from build123d import *

# Parameters (mm, degrees)
BOSS_EXTRUDE1_DEPTH = 2
BOSS_EXTRUDE2_DEPTH = 10
SKETCH7_R           = 3
SKETCH7_R_2         = 1.100094
SKETCH7_R_3         = 1.100095
SKETCH7_R_4         = 1.14540164
SKETCH7_R_5         = 1.100094267
BOSS_EXTRUDE3_DEPTH = 4
CUT_EXTRUDE1_DEPTH  = 3
FILLET2_R           = 1.3
CHAMFER1_SIZE       = 0.75
CHAMFER2_SIZE       = 0.5


with BuildPart() as part:
    # Sketch3 → Boss-Extrude1 (new body)
    with BuildSketch(Plane.XY):
        with BuildLine():
            Line((60.855233133, 23.823211938), (47.949977192, 24.377676222))
            Line((47.949977192, 24.377676222), (9.438001399, 18.932389733))
            ThreePointArc((9.438001399, 18.932389733), (7.157815869, 19.520564151), (5.962231275, 21.549300871))
            Line((5.962231275, 21.549300871), (-1.970708405, 77.995680607))
            ThreePointArc((-1.970708405, 77.995680607), (-1.383464331, 80.271537635), (0.639738461, 81.467794829))
            Line((0.639738461, 81.467794829), (38.699898469, 86.902208152))
            Line((38.699898469, 86.902208152), (38.171393284, 94.460167157))
            ThreePointArc((38.171393284, 94.460167157), (38.910984807, 96.683773594), (41.002517903, 97.740613468))
            Line((41.002517903, 97.740613468), (60.921819416, 99.276682226))
            Line((60.921819416, 99.276682226), (60.921819416, 103.721902307))
            ThreePointArc((60.921819416, 103.721902307), (61.804499235, 105.878127499), (63.945786912, 106.796450874))
            Line((63.945786912, 106.796450874), (83.059551455, 107.113531682))
            ThreePointArc((83.059551455, 107.113531682), (85.251859467, 106.245869167), (86.185286941, 104.080744272))
            Line((86.185286941, 104.080744272), (86.24375422, 99.780452187))
            Line((86.24375422, 99.780452187), (154.596820419, 99.780452187))
            ThreePointArc((154.596820419, 99.780452187), (156.771169517, 98.879807301), (157.671814403, 96.705458202))
            Line((157.671814403, 96.705458202), (157.671814403, 14.057773112))
            ThreePointArc((157.671814403, 14.057773112), (157.497078938, 13.035997261), (156.992732263, 12.130352296))
            Line((156.992732263, 12.130352296), (146.547659954, -0.852593653))
            ThreePointArc((146.547659954, -0.852593653), (144.453525054, -1.98521487), (142.178510717, -1.283401812))
            Line((142.178510717, -1.283401812), (127.110775499, 11.324099062))
            Line((127.110775499, 11.324099062), (110.204782414, 17.079131321))
            Line((110.204782414, 17.079131321), (91.635796855, 16.870620568))
            Line((91.635796855, 16.870620568), (72.085555936, 14.46343429))
            ThreePointArc((72.085555936, 14.46343429), (70.725838171, 14.602041008), (69.560483965, 15.316179508))
            Line((69.560483965, 15.316179508), (60.855233133, 23.823211938))
        make_face()
    extrude(amount=BOSS_EXTRUDE1_DEPTH)

    # Sketch4 → Boss-Extrude2 (add)
    with BuildSketch(Plane.XY):
        with BuildLine():
            Line((47.949977192, 24.377676222), (60.855233133, 23.823211938))
            Line((60.855233133, 23.823211938), (69.560483965, 15.316179508))
            ThreePointArc((69.560483965, 15.316179508), (70.725838171, 14.602041008), (72.085555936, 14.46343429))
            Line((72.085555936, 14.46343429), (91.635796855, 16.870620568))
            Line((91.635796855, 16.870620568), (110.204782414, 17.079131321))
            Line((110.204782414, 17.079131321), (127.110775499, 11.324099062))
            Line((127.110775499, 11.324099062), (142.178510717, -1.283401812))
            ThreePointArc((142.178510717, -1.283401812), (144.453525054, -1.98521487), (146.547659954, -0.852593653))
            Line((146.547659954, -0.852593653), (156.992732263, 12.130352296))
            ThreePointArc((156.992732263, 12.130352296), (157.497078938, 13.035997261), (157.671814403, 14.057773112))
            Line((157.671814403, 14.057773112), (157.671814403, 96.705458202))
            ThreePointArc((157.671814403, 96.705458202), (156.771169517, 98.879807301), (154.596820419, 99.780452187))
            Line((154.596820419, 99.780452187), (86.24375422, 99.780452187))
            Line((86.24375422, 99.780452187), (86.185286941, 104.080744272))
            ThreePointArc((86.185286941, 104.080744272), (85.251859467, 106.245869167), (83.059551455, 107.113531682))
            Line((83.059551455, 107.113531682), (63.945786912, 106.796450874))
            ThreePointArc((63.945786912, 106.796450874), (61.804499235, 105.878127499), (60.921819416, 103.721902307))
            Line((60.921819416, 103.721902307), (60.921819416, 99.276682226))
            Line((60.921819416, 99.276682226), (41.002517903, 97.740613468))
            ThreePointArc((41.002517903, 97.740613468), (38.910984807, 96.683773594), (38.171393284, 94.460167157))
            Line((38.171393284, 94.460167157), (38.699898469, 86.902208152))
            Line((38.699898469, 86.902208152), (0.639738461, 81.467794829))
            ThreePointArc((0.639738461, 81.467794829), (-1.383464331, 80.271537635), (-1.970708405, 77.995680607))
            Line((-1.970708405, 77.995680607), (5.962231275, 21.549300871))
            ThreePointArc((5.962231275, 21.549300871), (7.157815869, 19.520564151), (9.438001399, 18.932389733))
            Line((9.438001399, 18.932389733), (47.949977192, 24.377676222))
        make_face()
        with BuildLine():
            ThreePointArc((84.258355662, 98.692914663), (84.533669024, 98.04695842), (85.183308419, 97.780452187))
            Line((85.183308419, 97.780452187), (154.596820419, 97.780452187))
            ThreePointArc((154.596820419, 97.780452187), (155.356955955, 97.465593738), (155.671814403, 96.705458202))
            Line((155.671814403, 96.705458202), (155.671814403, 14.057773112))
            ThreePointArc((155.671814403, 14.057773112), (155.610734868, 13.70060696), (155.434438315, 13.38403486))
            Line((155.434438315, 13.38403486), (144.989366006, 0.401088911))
            ThreePointArc((144.989366006, 0.401088911), (144.257272174, 0.005133041), (143.461944249, 0.250481615))
            Line((143.461944249, 0.250481615), (128.108249423, 13.097251096))
            Line((128.108249423, 13.097251096), (110.524936275, 19.082852408))
            Line((110.524936275, 19.082852408), (91.501949272, 18.869243682))
            Line((91.501949272, 18.869243682), (71.841145237, 16.448443965))
            ThreePointArc((71.841145237, 16.448443965), (71.365754809, 16.496904248), (70.958318613, 16.74658445))
            Line((70.958318613, 16.74658445), (61.958856362, 25.54112911))
            ThreePointArc((61.958856362, 25.54112911), (61.679828995, 25.728441638), (61.352295386, 25.803701118))
            Line((61.352295386, 25.803701118), (47.852081394, 26.383727313))
            Line((47.852081394, 26.383727313), (9.158002316, 20.91269287))
            ThreePointArc((9.158002316, 20.91269287), (8.360780393, 21.118336461), (7.942767807, 21.827644264))
            Line((7.942767807, 21.827644264), (0.009828128, 78.274024))
            ThreePointArc((0.009828128, 78.274024), (0.215128769, 79.069664055), (0.922440855, 79.487875801))
            Line((0.922440855, 79.487875801), (39.972806225, 85.063675424))
            ThreePointArc((39.972806225, 85.063675424), (40.561555536, 85.398058084), (40.76480024, 86.043913413))
            Line((40.76480024, 86.043913413), (40.166521363, 94.599680421))
            ThreePointArc((40.166521363, 94.599680421), (40.425084652, 95.377059525), (41.156290542, 95.746533736))
            Line((41.156290542, 95.746533736), (62.067941403, 97.359127107))
            ThreePointArc((62.067941403, 97.359127107), (62.675544492, 97.652931317), (62.921819416, 98.281303094))
            Line((62.921819416, 98.281303094), (62.921819416, 103.721902307))
            ThreePointArc((62.921819416, 103.721902307), (63.230393236, 104.475691655), (63.978960617, 104.796726017))
            Line((63.978960617, 104.796726017), (83.09272516, 105.113806824))
            ThreePointArc((83.09272516, 105.113806824), (83.859148665, 104.810474928), (84.185471769, 104.053554549))
            Line((84.185471769, 104.053554549), (84.258355662, 98.692914663))
        make_face(mode=Mode.SUBTRACT)
    extrude(amount=BOSS_EXTRUDE2_DEPTH)

    # Sketch7 → Boss-Extrude3 (add)
    # profile 1 of 6: a face of its own
    with BuildSketch(Plane.XY):
        with Locations((25.178343626, 43.435558637)):
            Circle(SKETCH7_R)
        with Locations((25.178343626, 43.435558637)):
            Circle(SKETCH7_R_2, mode=Mode.SUBTRACT)
    # profile 2 of 6: a face of its own
    with BuildSketch(Plane.XY):
        with Locations((22.534055897, 62.250653675)):
            Circle(SKETCH7_R)
        with Locations((22.534055897, 62.250653675)):
            Circle(SKETCH7_R_2, mode=Mode.SUBTRACT)
    # profile 3 of 6: a face of its own
    with BuildSketch(Plane.XY):
        with Locations((63.99681822, 84.705447078)):
            Circle(SKETCH7_R)
        with Locations((63.99681822, 84.705447078)):
            Circle(SKETCH7_R_3, mode=Mode.SUBTRACT)
    # profile 4 of 6: a face of its own
    with BuildSketch(Plane.XY):
        with Locations((73.496822591, 41.005447941)):
            Circle(SKETCH7_R)
        with Locations((73.496822591, 41.005447941)):
            Circle(SKETCH7_R_3, mode=Mode.SUBTRACT)
    # profile 5 of 6: a face of its own
    with BuildSketch(Plane.XY):
        with Locations((124.796820928, 64.405450202)):
            Circle(SKETCH7_R)
        with Locations((124.796820928, 64.405450202)):
            Circle(SKETCH7_R_4, mode=Mode.SUBTRACT)
    # profile 6 of 6: a face of its own
    with BuildSketch(Plane.XY):
        with Locations((134.70931431, 21.546419059)):
            Circle(SKETCH7_R)
        with Locations((134.70931431, 21.546419059)):
            Circle(SKETCH7_R_5, mode=Mode.SUBTRACT)
    extrude(amount=BOSS_EXTRUDE3_DEPTH)

    # Sketch8 → Cut-Extrude1 (cut)
    with BuildSketch(Plane(origin=(157.671814403, 0, 0), x_dir=(0, 0, -1), z_dir=(1, 0, 0))):
        with BuildLine():
            Line((-2, 62.669458202), (-2, 52.669458202))
            ThreePointArc((-2, 52.669458202), (-4, 50.669458202), (-6, 52.669458202))
            Line((-6, 52.669458202), (-6, 62.669458202))
            ThreePointArc((-6, 62.669458202), (-4, 64.669458202), (-2, 62.669458202))
        make_face()
    extrude(amount=-CUT_EXTRUDE1_DEPTH, mode=Mode.SUBTRACT)

    # Fillet2
    fillet2_edges = [part.edges().sort_by_distance(p)[0] for p in [
        (65.207858549, 19.569695723, 0),
        (54.402605163, 24.10044408, 0),
        (28.693989296, 21.655032978, 0),
        (7.157815869, 19.520564151, 0),
        (1.995761435, 49.772490739, 0),
        (-1.383464331, 80.271537635, 0),
        (19.669818465, 84.18500149, 0),
        (38.435645877, 90.681187654, 0),
        (38.910984807, 96.683773594, 0),
        (50.962168659, 98.508647847, 0),
        (60.921819416, 101.499292266, 0),
        (61.804499235, 105.878127499, 0),
        (73.502669184, 106.954991278, 0),
        (85.251859467, 106.245869167, 0),
        (86.21452058, 101.930598229, 0),
        (120.420287319, 99.780452187, 0),
        (156.771169517, 98.879807301, 0),
        (157.671814403, 55.381615657, 0),
        (157.497078938, 13.035997261, 0),
        (151.770196108, 5.638879321, 0),
        (144.453525054, -1.98521487, 0),
        (134.644643108, 5.020348625, 0),
        (118.657778957, 14.201615191, 0),
        (100.920289635, 16.974875944, 0),
        (81.860676395, 15.667027429, 0),
        (70.725838171, 14.602041008, 0),
    ]]
    fillet(fillet2_edges, radius=FILLET2_R)

    # Chamfer1
    chamfer1_edges = [part.edges().sort_by_distance(p)[0] for p in [
        (70.725838171, 14.602041008, 10),
        (81.860676395, 15.667027429, 10),
        (100.920289635, 16.974875944, 10),
        (118.657778957, 14.201615191, 10),
        (134.644643108, 5.020348625, 10),
        (144.453525054, -1.98521487, 10),
        (151.770196108, 5.638879321, 10),
        (157.497078938, 13.035997261, 10),
        (157.671814403, 55.381615657, 10),
        (156.771169517, 98.879807301, 10),
        (120.420287319, 99.780452187, 10),
        (86.21452058, 101.930598229, 10),
        (85.251859467, 106.245869167, 10),
        (73.502669184, 106.954991278, 10),
        (61.804499235, 105.878127499, 10),
        (60.921819416, 101.499292266, 10),
        (50.962168659, 98.508647847, 10),
        (38.910984807, 96.683773594, 10),
        (38.435645877, 90.681187654, 10),
        (19.669818465, 84.18500149, 10),
        (-1.383464331, 80.271537635, 10),
        (1.995761435, 49.772490739, 10),
        (7.157815869, 19.520564151, 10),
        (28.693989296, 21.655032978, 10),
        (54.402605163, 24.10044408, 10),
        (65.207858549, 19.569695723, 10),
    ]]
    chamfer(chamfer1_edges, length=CHAMFER1_SIZE)

    # Chamfer2
    chamfer2_edges = [part.edges().sort_by_distance(p)[0] for p in [
        (133.609220043, 21.546419059, 4),
        (123.651419288, 64.405450202, 4),
        (72.396727591, 41.005447941, 4),
        (62.89672322, 84.705447078, 4),
        (21.433961897, 62.250653675, 4),
        (24.078249626, 43.435558637, 4),
    ]]
    chamfer(chamfer2_edges, length=CHAMFER2_SIZE)


solid = part.part
Verification items for the finished model (mm, model axes). A direction names the side the tool comes from. Coordinates: 2 decimals unless noted, no trailing zeros. Write each question's results on one line, items separated by ' | '.
Item 1: Gauge pin test, flat ends, axial feed: pin 1 (0.7 mm diameter, centred on x = 125.5, y = 65, fed in from +Z); pin 2 (1.8 mm diameter, centred on x = 124.5, y = 65.5, fed in from +Z); pin 3 (3 mm diameter, centred on x = 102, z = 6.5, fed in from +Y); pin 4 (5 mm diameter, centred on x = 94.5, y = 20.5, fed in from +Z). Record the tip position at first contact, or that the pin passes through.
Found:
pin 1: stops at z = 3.63 | pin 2: stops at z = 4 | pin 3: stops at y = 99.78 | pin 4: stops at z = 10
Item 2: Mould release check, pull along X, two halves, no side actions. Record for faces 4 (the face through (156.4, 98.47, 9.8)), 5 (the face through (71.286, 43.033, 2.986)), 6 (the face through (61.781, 105.854, 5.219)): +X half, -X half, draft (parallel to the pull), parting line (faces both ways), or undercut.
Found:
face 4: +X half | face 5: undercut | face 6: -X half
Item 3: Material ranges on L1, parallel to Y at x = 108.5, z = 7.75; L2, parallel to X at y = 35.5, z = 5.25; L3, parallel to Y at x = 49, z = 3, recorded low to high.
Found:
L1: y = 17.06 to 19.06, 97.78 to 99.78 | L2: x = 4 to 6.02, 155.67 to 157.67 | L3: y = 24.33 to 26.33, 96.35 to 98.36
Item 4: Tool access check on faces 1 (the face through (40.47, 90.26, 5.94)), 2 (the face through (28.4, 22, 9.63)), 3 (the face through (81.998, 15.684, 5.219)). Record the directions out of +Z, -Z, +X, -X, +Y, -Y that give a thin tool (end or side, any length) a straight path to the whole face; none if there is none.
Found:
face 1: +Z | face 2: +Z, -Y | face 3: +Z, -Z, -Y
